Geometry: final body of the model. Coordinates: model frame, mm. Give positions to 0.01 mm unless a question says otherwise; leave off trailing zeros. Write each loop counter-clockwise with the first axis right and the second up, starting at its lowest first coordinate (ties: lowest second). Pieces come first, ordered by that corner, then holes. Notation, with made-up numbers: (43.25, 37.25) - (60.25, 37.25) arc R29 ccw to (60.25, 66.25) - close; hole circle Ø10 at (-37, 27). An arc over 180 degrees is marked (long way). Return JSON: item names as keys, results as strings.
from build123d import *

# Parameters (mm, degrees)
F0_R     = 1.5875
F0_W     = 159.1020785272
F0_H     = 25.4
F1_DEPTH = 2.9718


# Not quite as in the source:
# - a feature names something its author has since deleted; it is built from what else it names


with BuildPart() as f1:
    # F0 (on Front) → F1 (new body)
    with BuildSketch(Plane.XZ):
        Polygon((-134.1324669933, 51.0296365122), (-134.1324669933, 54.0014365122), (-136.6724669933, 54.0014365122), (-136.6724669933, -22.1985634878), (-134.1324669933, -22.1985634878), (-134.1324669933, -19.2267634878), align=None)
        with BuildLine():
            Line((-130.6399669933, 51.0296365122), (-134.1324669933, 51.0296365122))
            Line((-134.1324669933, 51.0296365122), (-134.1324669933, -19.2267634878))
            Line((-134.1324669933, -19.2267634878), (-130.6399669933, -19.2267634878))
            Line((-130.6399669933, -19.2267634878), (-130.6399669933, -13.8642910361))
            Line((-130.6399669933, -13.8642910361), (-133.683725667, -13.8642910361))
            Line((-133.683725667, -13.8642910361), (-133.683725667, -10.6892910361))
            Line((-133.683725667, -10.6892910361), (-130.6399669933, -10.6892910361))
            Line((-130.6399669933, -10.6892910361), (-130.6399669933, -9.4985634878))
            Line((-130.6399669933, -9.4985634878), (-127.4649669933, -9.4985634878))
            Line((-127.4649669933, -9.4985634878), (-127.4649669933, -10.6892910361))
            Line((-127.4649669933, -10.6892910361), (-124.158725667, -10.6892910361))
            Line((-124.158725667, -10.6892910361), (-124.158725667, -13.8642910361))
            Line((-124.158725667, -13.8642910361), (-127.4649669933, -13.8642910361))
            Line((-127.4649669933, -13.8642910361), (-127.4649669933, -19.2267634878))
            Line((-127.4649669933, -19.2267634878), (-120.5434669933, -19.2267634878))
            Line((-120.5434669933, -19.2267634878), (-120.5434669933, -12.0385634878))
            Line((-120.5434669933, -12.0385634878), (-51.9634669933, -12.0385634878))
            Line((-51.9634669933, -12.0385634878), (-51.9634669933, -19.2267634878))
            Line((-51.9634669933, -19.2267634878), (-40.7874669933, -19.2267634878))
            Line((-40.7874669933, -19.2267634878), (-40.7874669933, -13.650716418))
            Line((-40.7874669933, -13.650716418), (-43.0311936414, -13.650716418))
            Line((-43.0311936414, -13.650716418), (-43.0311936414, -10.475716418))
            Line((-43.0311936414, -10.475716418), (-40.7874669933, -10.475716418))
            Line((-40.7874669933, -10.475716418), (-40.7874669933, -9.4985634878))
            Line((-40.7874669933, -9.4985634878), (-37.6124669933, -9.4985634878))
            Line((-37.6124669933, -9.4985634878), (-37.6124669933, -10.475716418))
            Line((-37.6124669933, -10.475716418), (-35.4111936414, -10.475716418))
            Line((-35.4111936414, -10.475716418), (-35.4111936414, -13.650716418))
            Line((-35.4111936414, -13.650716418), (-37.6124669933, -13.650716418))
            Line((-37.6124669933, -13.650716418), (-37.6124669933, -19.2267634878))
            Line((-37.6124669933, -19.2267634878), (-32.5324669933, -19.2267634878))
            Line((-32.5324669933, -19.2267634878), (-32.5324669933, -22.1985634878))
            Line((-32.5324669933, -22.1985634878), (-7.1324669933, -22.1985634878))
            Line((-7.1324669933, -22.1985634878), (-7.1324669933, -19.2267634878))
            Line((-7.1324669933, -19.2267634878), (3.9800330067, -19.2267634878))
            Line((3.9800330067, -19.2267634878), (3.9800330067, -13.4051909164))
            Line((3.9800330067, -13.4051909164), (1.6932926612, -13.4051909164))
            Line((1.6932926612, -13.4051909164), (1.6932926612, -10.2301909164))
            Line((1.6932926612, -10.2301909164), (3.9800330067, -10.2301909164))
            Line((3.9800330067, -10.2301909164), (3.9800330067, -9.4985634878))
            Line((3.9800330067, -9.4985634878), (7.1550330067, -9.4985634878))
            Line((7.1550330067, -9.4985634878), (7.1550330067, -10.2301909164))
            Line((7.1550330067, -10.2301909164), (9.3132926612, -10.2301909164))
            Line((9.3132926612, -10.2301909164), (9.3132926612, -13.4051909164))
            Line((9.3132926612, -13.4051909164), (7.1550330067, -13.4051909164))
            Line((7.1550330067, -13.4051909164), (7.1550330067, -19.2267634878))
            Line((7.1550330067, -19.2267634878), (18.2675330067, -19.2267634878))
            Line((18.2675330067, -19.2267634878), (18.2675330067, -22.1985634878))
            Line((18.2675330067, -22.1985634878), (43.6675330067, -22.1985634878))
            Line((43.6675330067, -22.1985634878), (43.6675330067, -19.2267634878))
            Line((43.6675330067, -19.2267634878), (54.7800330067, -19.2267634878))
            Line((54.7800330067, -19.2267634878), (54.7800330067, -13.545062393))
            Line((54.7800330067, -13.545062393), (52.6228938252, -13.545062393))
            Line((52.6228938252, -13.545062393), (52.6228938252, -10.370062393))
            Line((52.6228938252, -10.370062393), (54.7800330067, -10.370062393))
            Line((54.7800330067, -10.370062393), (54.7800330067, -9.4985634878))
            Line((54.7800330067, -9.4985634878), (57.9550330067, -9.4985634878))
            Line((57.9550330067, -9.4985634878), (57.9550330067, -10.370062393))
            Line((57.9550330067, -10.370062393), (60.2428938252, -10.370062393))
            Line((60.2428938252, -10.370062393), (60.2428938252, -13.545062393))
            Line((60.2428938252, -13.545062393), (57.9550330067, -13.545062393))
            Line((57.9550330067, -13.545062393), (57.9550330067, -19.2267634878))
            Line((57.9550330067, -19.2267634878), (69.0675330067, -19.2267634878))
            Line((69.0675330067, -19.2267634878), (69.0675330067, -22.1985634878))
            Line((69.0675330067, -22.1985634878), (94.4675330067, -22.1985634878))
            add(Edge.make_bspline(
                [(94.4675330067, 15.9014365122), (33.4221309805, -6.5926179945), (67.8742191577, 4.6496394366), (94.4675330067, -22.1985634878)],
                knots=[0, 0, 0, 0, 38.1, 38.1, 38.1, 38.1], degree=3))
            add(Edge.make_bspline(
                [(94.4675330067, 54.0014365122), (67.8547954941, 24.2413681328), (34.147437551, 33.6619180903), (94.4675330067, 15.9014365122)],
                knots=[0, 0, 0, 0, 38.1, 38.1, 38.1, 38.1], degree=3))
            Line((94.4675330067, 54.0014365122), (69.0675330067, 54.0014365122))
            Line((69.0675330067, 54.0014365122), (69.0675330067, 51.0296365122))
            Line((69.0675330067, 51.0296365122), (57.9550330067, 51.0296365122))
            Line((57.9550330067, 51.0296365122), (57.9550330067, 45.263365978))
            Line((57.9550330067, 45.263365978), (60.3188354051, 45.263365978))
            Line((60.3188354051, 45.263365978), (60.3188354051, 42.088365978))
            Line((60.3188354051, 42.088365978), (57.9550330067, 42.088365978))
            Line((57.9550330067, 42.088365978), (57.9550330067, 41.3014365122))
            Line((57.9550330067, 41.3014365122), (54.7800330067, 41.3014365122))
            Line((54.7800330067, 41.3014365122), (54.7800330067, 42.088365978))
            Line((54.7800330067, 42.088365978), (52.6988354051, 42.088365978))
            Line((52.6988354051, 42.088365978), (52.6988354051, 45.263365978))
            Line((52.6988354051, 45.263365978), (54.7800330067, 45.263365978))
            Line((54.7800330067, 45.263365978), (54.7800330067, 51.0296365122))
            Line((54.7800330067, 51.0296365122), (43.6675330067, 51.0296365122))
            Line((43.6675330067, 51.0296365122), (43.6675330067, 54.0014365122))
            Line((43.6675330067, 54.0014365122), (18.2675330067, 54.0014365122))
            Line((18.2675330067, 54.0014365122), (18.2675330067, 51.0296365122))
            Line((18.2675330067, 51.0296365122), (7.1550330067, 51.0296365122))
            Line((7.1550330067, 51.0296365122), (7.1550330067, 45.1199758291))
            Line((7.1550330067, 45.1199758291), (9.3046905002, 45.1199758291))
            Line((9.3046905002, 45.1199758291), (9.3046905002, 41.9449758291))
            Line((9.3046905002, 41.9449758291), (7.1550330067, 41.9449758291))
            Line((7.1550330067, 41.9449758291), (7.1550330067, 41.3014365122))
            Line((7.1550330067, 41.3014365122), (3.9800330067, 41.3014365122))
            Line((3.9800330067, 41.3014365122), (3.9800330067, 41.9449758291))
            Line((3.9800330067, 41.9449758291), (1.6846905002, 41.9449758291))
            Line((1.6846905002, 41.9449758291), (1.6846905002, 45.1199758291))
            Line((1.6846905002, 45.1199758291), (3.9800330067, 45.1199758291))
            Line((3.9800330067, 45.1199758291), (3.9800330067, 51.0296365122))
            Line((3.9800330067, 51.0296365122), (-7.1324669933, 51.0296365122))
            Line((-7.1324669933, 51.0296365122), (-7.1324669933, 54.0014365122))
            Line((-7.1324669933, 54.0014365122), (-32.5324669933, 54.0014365122))
            Line((-32.5324669933, 54.0014365122), (-32.5324669933, 51.0296365122))
            Line((-32.5324669933, 51.0296365122), (-37.6124669933, 51.0296365122))
            Line((-37.6124669933, 51.0296365122), (-37.6124669933, 45.4024068505))
            Line((-37.6124669933, 45.4024068505), (-35.3795323992, 45.4024068505))
            Line((-35.3795323992, 45.4024068505), (-35.3795323992, 42.2274068505))
            Line((-35.3795323992, 42.2274068505), (-37.6124669933, 42.2274068505))
            Line((-37.6124669933, 42.2274068505), (-37.6124669933, 41.3014365122))
            Line((-37.6124669933, 41.3014365122), (-40.7874669933, 41.3014365122))
            Line((-40.7874669933, 41.3014365122), (-40.7874669933, 42.2274068505))
            Line((-40.7874669933, 42.2274068505), (-42.9995323992, 42.2274068505))
            Line((-42.9995323992, 42.2274068505), (-42.9995323992, 45.4024068505))
            Line((-42.9995323992, 45.4024068505), (-40.7874669933, 45.4024068505))
            Line((-40.7874669933, 45.4024068505), (-40.7874669933, 51.0296365122))
            Line((-40.7874669933, 51.0296365122), (-51.9634669933, 51.0296365122))
            Line((-51.9634669933, 51.0296365122), (-51.9634669933, 43.8414365122))
            Line((-51.9634669933, 43.8414365122), (-120.5434669933, 43.8414365122))
            Line((-120.5434669933, 43.8414365122), (-120.5434669933, 51.0296365122))
            Line((-120.5434669933, 51.0296365122), (-127.4649669933, 51.0296365122))
            Line((-127.4649669933, 51.0296365122), (-127.4649669933, 45.3533373266))
            Line((-127.4649669933, 45.3533373266), (-124.5652367949, 45.3533373266))
            Line((-124.5652367949, 45.3533373266), (-124.5652367949, 42.1783373266))
            Line((-124.5652367949, 42.1783373266), (-127.4649669933, 42.1783373266))
            Line((-127.4649669933, 42.1783373266), (-127.4649669933, 41.3014365122))
            Line((-127.4649669933, 41.3014365122), (-130.6399669933, 41.3014365122))
            Line((-130.6399669933, 41.3014365122), (-130.6399669933, 42.1783373266))
            Line((-130.6399669933, 42.1783373266), (-134.0902367949, 42.1783373266))
            Line((-134.0902367949, 42.1783373266), (-134.0902367949, 45.3533373266))
            Line((-134.0902367949, 45.3533373266), (-130.6399669933, 45.3533373266))
            Line((-130.6399669933, 45.3533373266), (-130.6399669933, 51.0296365122))
        make_face()
        with Locations((-95.7784669933, -3.1485634878)):
            Circle(F0_R, mode=Mode.SUBTRACT)
        with BuildLine():
            ThreePointArc((-75.1409669933, -3.1485634878), (-76.7284669933, -4.7360634878), (-78.3159669933, -3.1485634878))
            ThreePointArc((-78.3159669933, -3.1485634878), (-76.7284669933, -1.5610634878), (-75.1409669933, -3.1485634878))
        make_face(mode=Mode.SUBTRACT)
        with Locations((8.7425330067, -3.1485634878)):
            Circle(F0_R, mode=Mode.SUBTRACT)
        with BuildLine():
            ThreePointArc((29.3800330067, -3.1485634878), (27.7925330067, -4.7360634878), (26.2050330067, -3.1485634878))
            ThreePointArc((26.2050330067, -3.1485634878), (27.7925330067, -1.5610634878), (29.3800330067, -3.1485634878))
        make_face(mode=Mode.SUBTRACT)
        with Locations((-29.1814277297, 15.9014365122)):
            Rectangle(F0_W, F0_H, mode=Mode.SUBTRACT)
        with Locations((-95.7784669933, 34.9514365122)):
            Circle(F0_R, mode=Mode.SUBTRACT)
        with BuildLine():
            ThreePointArc((-75.1409669933, 34.9514365122), (-76.7284669933, 33.3639365122), (-78.3159669933, 34.9514365122))
            ThreePointArc((-78.3159669933, 34.9514365122), (-76.7284669933, 36.5389365122), (-75.1409669933, 34.9514365122))
        make_face(mode=Mode.SUBTRACT)
        with Locations((8.7425330067, 34.9514365122)):
            Circle(F0_R, mode=Mode.SUBTRACT)
        with BuildLine():
            ThreePointArc((29.3800330067, 34.9514365122), (27.7925330067, 33.3639365122), (26.2050330067, 34.9514365122))
            ThreePointArc((26.2050330067, 34.9514365122), (27.7925330067, 36.5389365122), (29.3800330067, 34.9514365122))
        make_face(mode=Mode.SUBTRACT)
        with Locations((-29.1814277297, 15.9014365122)):
            Rectangle(F0_W, F0_H)
    extrude(amount=F1_DEPTH)


solid = f1.part
Q1. Section query B-B, the plane x = -111. Return the cut outline in (y, z).
Answer key:
{"outline": "(-2.97, -12.04) - (0, -12.04) - (0, 43.84) - (-2.97, 43.84) - close"}
Q2. Pin query (flat end, axial travel): P1, Ø0.9, axis at y = -2, z = -15.5, coming from the +X side; P2, Ø1.5, axis at x = -131.5, y = -1.5, coming from the +Z side; P3, Ø1.5, axis at x = -133, y = -1.5, coming from the -Z side. Return the tip coordinate at first contact, or that it passes through.
Answer key:
{"P1": "stops at x = 87.34", "P2": "stops at z = 51.03", "P3": "stops at z = -19.23"}
Q3. Section query A-A, the plane x = 76. Count the separate pieces of the cut face and the enclosed holes in it, plus the area to 3 significant figures.
Answer key:
{"separate pieces": "3", "enclosed holes": "0", "area": "122 mm^2"}
Q4. Material intervals for probe 1 along Z at (x, y) = (-37, -1.2); probe 2 along X at (y, z) = (-0.7, -17); probe 3 along Z at (x, y) = (63.5, -1.5), sorted ascending. Write a range as [from, to].
Answer key:
{"probe 1": "z = [-19.23, -13.65], [-10.48, 42.23], [45.4, 51.03]", "probe 2": "x = [-136.67, -130.64], [-127.46, -120.54], [-51.96, -40.79], [-37.61, 3.98], [7.16, 54.78], [57.96, 88.68]", "probe 3": "z = [-19.23, -2.71], [3.43, 25.98], [31.62, 51.03]"}
